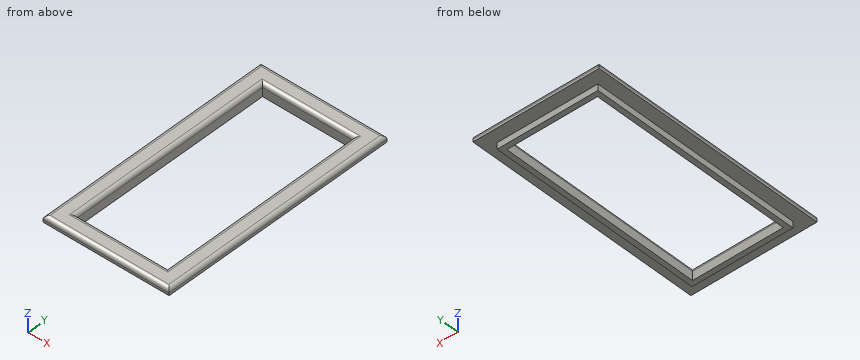
from build123d import *

# Parameters (mm, degrees)
CROQUIS1_W              = 40
CROQUIS1_H              = 85
CROQUIS1_W_2            = 36
CROQUIS1_H_2            = 81
SALIENTE_EXTRUIR2_DEPTH = 2.5
CROQUIS2_W              = 50
CROQUIS2_H              = 95
CROQUIS2_W_2            = 40
CROQUIS2_H_2            = 85
SALIENTE_EXTRUIR3_DEPTH = 2.5
REDONDEO1_R             = 1.5


with BuildPart() as part:
    # Croquis1 → Saliente-Extruir2 (new, symmetric)
    with BuildSketch(Plane.XY):
        Rectangle(CROQUIS1_W, CROQUIS1_H)
        Rectangle(CROQUIS1_W_2, CROQUIS1_H_2, mode=Mode.SUBTRACT)
    extrude(amount=SALIENTE_EXTRUIR2_DEPTH, both=True)

    # Croquis2 → Saliente-Extruir3 (add)
    with BuildSketch(Plane.XY):
        Rectangle(CROQUIS2_W, CROQUIS2_H)
        Rectangle(CROQUIS2_W_2, CROQUIS2_H_2, mode=Mode.SUBTRACT)
    extrude(amount=SALIENTE_EXTRUIR3_DEPTH)

    # Redondeo1
    redondeo1_edges = [part.edges().sort_by_distance(p)[0] for p in [
        (-18, 0, 2.5),
        (0, -40.5, 2.5),
        (18, 0, 2.5),
        (0, 40.5, 2.5),
        (-25, 0, 2.5),
        (0, -47.5, 2.5),
        (25, 0, 2.5),
        (0, 47.5, 2.5),
    ]]
    fillet(redondeo1_edges, radius=REDONDEO1_R)


solid = part.part
Build history of the part. All positions in model axes, mm. Coordinates: 2 decimals unless noted, no trailing zeros. Write each loop counter-clockwise with the first axis right and the second up, starting at its lowest first coordinate (ties: lowest second). Pieces come first, ordered by that corner, then holes.
(1) Pin check, flat tips, straight feed: pin 1 Ø1.2 at (x, z) = (-4, -1) entering from +Y; pin 2 Ø2 at (x, y) = (16, -11.5) entering from -Z; pin 3 Ø1.2 at (y, z) = (18.5, -1) entering from -X; pin 4 Ø0.8 at (y, z) = (-15, -0.5) entering from +X. Stop position of each tip, or through.
(2) Cut at C-C on x = 16. List the corners of the cut face in (y, z).
(3) Cut at A-A on y = 28.5. List the corners of the cut face in (x, z), and give its area (3 significant figures).
(4) Cut at D-D on x = -21. List the corners of the cut face in (y, z).
(5) Drill centre lines: line 1 (Y direction, x = 4.5, z = -1.9); line 2 (Y direction, x = -17, z = 1.05); line 3 (X direction, y = 16, z = -0.6). Where is each one in solid material? Low to high.
(6) Cut at B-B on z = -1.2. List the corners of the cut face in (x, y), and give its area (3 significant figures).
Working result:
1. pin 1: stops at y = 42.5
1. pin 2: passes through
1. pin 3: stops at x = -20
1. pin 4: stops at x = 20
2. outline: (-47.5, 0) - (-42.5, 0) - (-42.5, -2.5) - (-40.5, -2.5) - (-40.5, 1) arc R1.5 ccw to (-42, 2.5) - (-46, 2.5) arc R1.5 ccw to (-47.5, 1) - close; (40.5, -2.5) - (42.5, -2.5) - (42.5, 0) - (47.5, 0) - (47.5, 1) arc R1.5 ccw to (46, 2.5) - (42, 2.5) arc R1.5 ccw to (40.5, 1) - close
3. outline: (-25, 0) - (-20, 0) - (-20, -2.5) - (-18, -2.5) - (-18, 1) arc R1.5 ccw to (-19.5, 2.5) - (-23.5, 2.5) arc R1.5 ccw to (-25, 1) - close; (18, -2.5) - (20, -2.5) - (20, 0) - (25, 0) - (25, 1) arc R1.5 ccw to (23.5, 2.5) - (19.5, 2.5) arc R1.5 ccw to (18, 1) - close
3. area: 43.1 mm2
4. outline: (-47.5, 0) - (47.5, 0) - (47.5, 1) arc R1.5 ccw to (46, 2.5) - (-46, 2.5) arc R1.5 ccw to (-47.5, 1) - close
5. line 1: y = -42.5 to -40.5, 40.5 to 42.5
5. line 2: y = -47.5 to -40.5, 40.5 to 47.5
5. line 3: x = -20 to -18, 18 to 20
6. outline: (-20, -42.5) - (20, -42.5) - (20, 42.5) - (-20, 42.5) - close; hole (-18, -40.5) - (18, -40.5) - (18, 40.5) - (-18, 40.5) - close
6. area: 484 mm2
